Input: dimensioned drawing with shaded views. Units: mm. Origin: part minimum x, y, z. A direction names the side the tool comes from. Coordinates: 2 decimals unless noted, no trailing zeros. Write each loop counter-clockwise with the first axis right and the second up, starting at its lowest first coordinate (ties: lowest second). Pieces come first, ordered by that corner, then holes. Notation, with made-up numbers: M 9,-3 L 50,-3 A20 ccw 50,7 Z; hole C 72,83.25 d5. An arc over 180 degrees is marked long. Use one line per item in the form item = value.
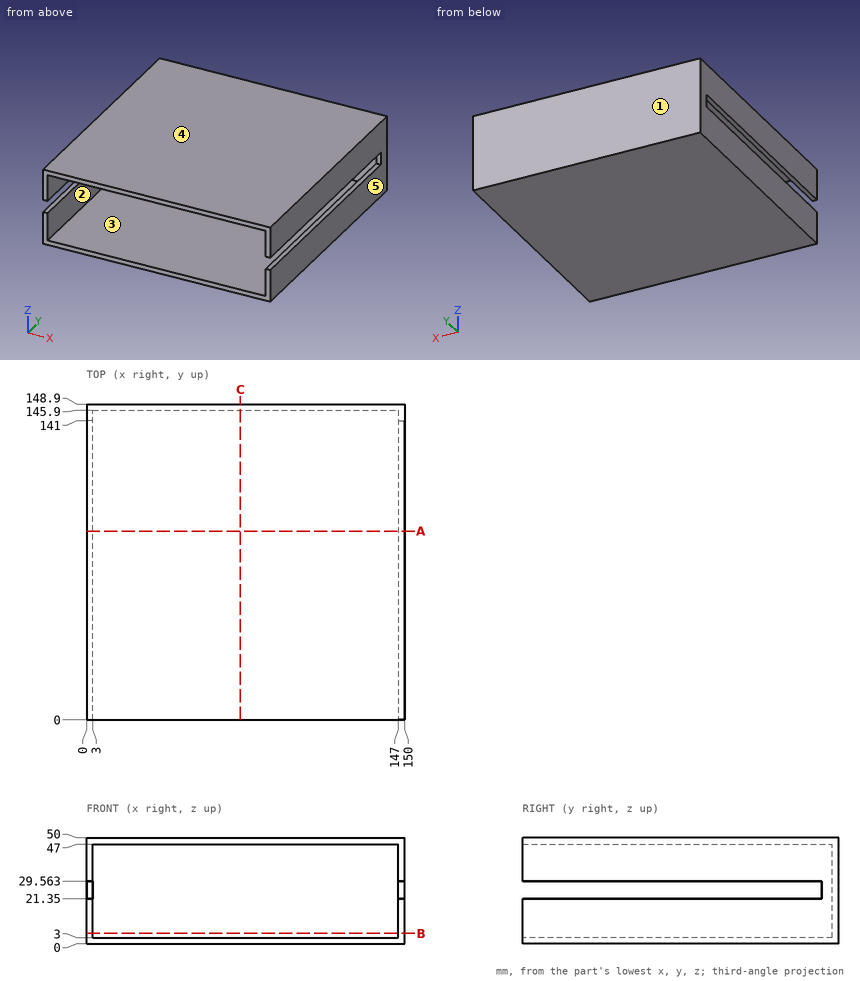
(1) First-contact query: pin 1 Ø10 at (x, z) = (98, 24) entering from -Y; pin 2 Ø2.5 at (x, z) = (2, 26.5) entering from -Y. Flat tips, straight axial feed; report the tip coordinate or a pass-through.
Computed:
pin_1 = 145.9
pin_2 = 141
(2) Section query B-B on z = 5. Return the cut outline in (x, y).
Computed:
outline = M 0,0 L 3,0 L 3,145.9 L 147,145.9 L 147,0 L 150,0 L 150,148.9 L 0,148.9 Z
(3) Section query A-A on y = 89. Return the cut outline in (x, z).
Computed:
outline = M 0,0 L 150,0 L 150,21.35 L 147,21.35 L 147,3 L 3,3 L 3,21.35 L 0,21.35 Z; M 0,29.56 L 3,29.56 L 3,47 L 147,47 L 147,29.56 L 150,29.56 L 150,50 L 0,50 Z
(4) Pull-direction query (Z, two-part tool) for the marked faces 3, 4 and 5; classes: pulls with the +Z half, pulls with the -Z half, needs draft (parallel to the pull), parting line crosses it, or undercut.
Computed:
face_3 = undercut
face_4 = pulls with the +Z half
face_5 = needs draft
(5) Section query C-C on x = 72.5. Return the cut outline in (y, z).
Computed:
outline = M 0,0 L 148.9,0 L 148.9,50 L 0,50 L 0,47 L 145.9,47 L 145.9,3 L 0,3 Z
(6) Set-up query: the marked faces 1 and 2. Return all of +Z, -Z, +X, -X, +Y, -Y with unobstructed straight access to the full face (end or side cutting, diameter ignored); none if empty.
Computed:
face_1 = +Z, -Z, +X, -X, +Y
face_2 = -Y
(7) Line query: probe 1 along Z at (x, y) = (62.5, 135); probe 2 along X at (y, z) = (72, 10.5); probe 3 along Y at (x, z) = (107, 35.5). Output: solid intervals per line, ascending.
Computed:
probe_1 = 0 to 3, 47 to 50
probe_2 = 0 to 3, 147 to 150
probe_3 = 145.9 to 148.9
